from build123d import *

# Parameters (mm, degrees)
CUT_EXTRUDE1_DEPTH = 14.329999999999998
CUT_EXTRUDE2_START = -14.33
CUT_EXTRUDE2_DEPTH = 3.12
SKETCH3_R          = 8.878997023709873
CUT_EXTRUDE3_DEPTH = 10
CIRPATTERN1_COUNT  = 6


with BuildPart() as part:
    # Sketch1 → Revolve1 (revolve)
    with BuildSketch(Plane.XY, mode=Mode.PRIVATE) as revolve1_sk:
        with BuildLine():
            Line((0, 0), (-50.4860955695321, 0))
            add(Edge.make_bspline(
                [(-52.01874999999999, 7.99999999999998), (-50.16036303063599, 4.2035390390822025), (-50.4860955695321, 0)],
                knots=[0, 0, 0, 1, 1, 1], degree=2))
            ThreePointArc((-52.01874999999999, 7.99999999999998), (-51.43296356237308, 9.414213562373089), (-50.018749999999976, 9.999999999999993))
            Line((-50.018749999999976, 9.999999999999993), (-47.018750000000004, 9.999999999999993))
            ThreePointArc((-47.018750000000004, 9.999999999999993), (-45.6045364376269, 9.414213562373089), (-45.01874999999999, 7.99999999999998))
            Line((-45.01874999999999, 7.99999999999998), (-45.01874999999999, 6.499999999999996))
            Line((-45.01874999999999, 6.499999999999996), (-5.018749999999988, 6.499999999999994))
            add(Edge.make_bspline(
                [(-5.018749999999988, 6.499999999999994), (5.878733880748029, 4.24822033263461), (16.98125000000001, 5.000000000000002)],
                knots=[0, 0, 0, 1, 1, 1], degree=2))
            Line((16.98125000000001, 5.000000000000002), (26.981250000000014, 5.000000000000003))
            Line((26.981250000000014, 5.000000000000003), (44.98125000000002, 3.0000000000000058))
            Line((44.98125000000002, 3.0000000000000058), (44.98125000000002, 5.51e-15))
            Line((44.98125000000002, 5.51e-15), (0, 0))
        make_face()
    revolve(revolve1_sk.sketch.rotate(Axis((-50.4860955695321, 0, 0), (1, 0, 0)), 90), axis=Axis((-50.4860955695321, 0, 0), (1, 0, 0)))

    # Sketch2 → Cut-Extrude1 (cut)
    with BuildSketch(Plane(origin=(44.98125000000002, 0, 0), x_dir=(0, 0, -1), z_dir=(1, 0, 0))):
        with BuildLine():
            ThreePointArc((1.0698598038995577, 0.6749999999999999), (8e-17, 1.265), (-1.0698598038995573, 0.6750000000000003))
            Line((-1.0698598038995575, 0.675), (1.0698598038995575, 0.675))
        make_face()
        with BuildLine():
            Line((1.0698598038995575, -0.675), (-1.0698598038995575, -0.675))
            ThreePointArc((-1.0698598038995577, -0.6749999999999999), (-2.3e-16, -1.265), (1.0698598038995577, -0.6749999999999998))
        make_face()
        with BuildLine():
            ThreePointArc((-1.0698598038995573, 0.6750000000000003), (-1.265, 1.5e-16), (-1.0698598038995577, -0.6749999999999999))
            Line((-1.0698598038995575, -0.675), (1.0698598038995575, -0.675))
            ThreePointArc((1.0698598038995577, -0.6749999999999998), (1.2152361194296644, -0.3513206143019937), (1.265, -3.1e-16))
            ThreePointArc((1.265, 0), (1.2152361194296646, 0.351320614301993), (1.0698598038995577, 0.6749999999999999))
            Line((1.0698598038995575, 0.675), (-1.0698598038995575, 0.675))
        make_face()
    extrude(amount=-CUT_EXTRUDE1_DEPTH, mode=Mode.SUBTRACT)

    # Sketch2<3> → Cut-Extrude2 (cut)
    with BuildSketch(Plane(origin=(44.98125000000002, 0, 0), x_dir=(0, 0, -1), z_dir=(1, 0, 0)).offset(CUT_EXTRUDE2_START)):
        with BuildLine():
            ThreePointArc((-1.0698598038995573, 0.6750000000000003), (-1.265, 1.5e-16), (-1.0698598038995577, -0.6749999999999999))
            Line((-1.0698598038995575, -0.675), (1.0698598038995575, -0.675))
            ThreePointArc((1.0698598038995577, -0.6749999999999998), (1.2152361194296644, -0.3513206143019937), (1.265, -3.1e-16))
            ThreePointArc((1.265, 0), (1.2152361194296646, 0.351320614301993), (1.0698598038995577, 0.6749999999999999))
            Line((1.0698598038995575, 0.675), (-1.0698598038995575, 0.675))
        make_face()
    extrude(amount=-CUT_EXTRUDE2_DEPTH, mode=Mode.SUBTRACT)

    # Sketch3 → Cut-Extrude3 (cut)
    with BuildSketch(Plane(origin=(-45.01874999999999, 0, 0), x_dir=(0, 0, -1), z_dir=(1, 0, 0))):
        with Locations((16.727573230529202, -6.401670880419097)):
            Circle(SKETCH3_R)
    cut_extrude3 = extrude(amount=-CUT_EXTRUDE3_DEPTH, mode=Mode.SUBTRACT)

    # CirPattern1: Cut-Extrude3 ×6 about axis
    cirpattern1_axis = Axis((0, -1.97e-14, 8.2e-15), (1, 0, 0))
    for i in range(1, CIRPATTERN1_COUNT):
        add(cut_extrude3.rotate(cirpattern1_axis, i * 360 / CIRPATTERN1_COUNT), mode=Mode.SUBTRACT)


solid = part.part
The model under review builds one solid part; all positions refer to its coordinate system, in mm. A direction names the side the tool comes from. Coordinates: 2 decimals unless noted, no trailing zeros. Write each loop counter-clockwise with the first axis right and the second up, starting at its lowest first coordinate (ties: lowest second). Pieces come first, ordered by that corner, then holes. Notation, with made-up numbers: (47.5, 9.25) - (105.5, 9.25) arc R11 ccw to (105.5, 18.25) - close; hole circle Ø4 at (49, 64.25). An arc over 180 degrees is marked (long way). Answer as a JSON object with one key per item and string values. Group by question number.
1. Add section A-A (x = 19). Give the boundary of the cut face in (y, z).
2. To check wall thickness, follow probe 1 along X at (y, z) = (5.75, -5.75); probe 2 along Y at (x, z) = (37, 0) (3 decimals); probe 3 along Y at (x, z) = (32, 0) (3 decimals). State the ranges of each line that lie inside material, in increasing order.
3. Machinability: for faces 4 (the face through (-45.019, -7, 0)), 5 (the face through (-48.47, 3.19, 8.45)), which of the approach directions +Z, -Z, +X, -X, +Y, -Y give a long, thin tool a straight path to every point of the face, cutting with its end or side? Answer none if there is none.
4. Clearance check with flat-ended pins moving along their axes: pin 1 Ø1 at (x, z) = (-36.5, 6.5) entering from -Y; pin 2 Ø10 at (x, y) = (-0.5, 2) entering from -Z; pin 3 Ø1.5 at (y, z) = (0, 0) entering from +X. State where each tip first meets the part, or that it passes through.
5. Add section B-B (x = 39). Give the boundary of the cut face in (y, z) (3 decimals), plus the area to 3 significant figures.
6. Mouldability with a two-part tool opening along Y and no side actions: class faces 1 (the face through (-48.474, 8.912, 1.464)), 2 (the face through (-48.474, -8.912, -1.464)), 3 (the face through (29, 0.675, 0)) as pulls with the +Y half, pulls with the -Y half, needs draft (parallel to the pull), parting line crosses it, or undercut.
Findings:
{
 "1": {"outline": "circle Ø10 at (0, 0)"},
 "2": {"probe 1": "-52.01 to -45.02", "probe 2": "-3.887 to -1.265, 1.265 to 3.887", "probe 3": "-4.442 to -1.265, 1.265 to 4.442"},
 "3": {"face 4": "+X", "face 5": "+Z, +X, -X, +Y"},
 "4": {"pin 1": "y = -2.5", "pin 2": "z = -6.5", "pin 3": "x = 30.65"},
 "5": {"outline": "circle Ø7.329 at (0, 0); hole circle Ø2.53 at (0, 0)", "area": "37.2 mm²"},
 "6": {"face 1": "pulls with the +Y half", "face 2": "pulls with the -Y half", "face 3": "undercut"}
}
